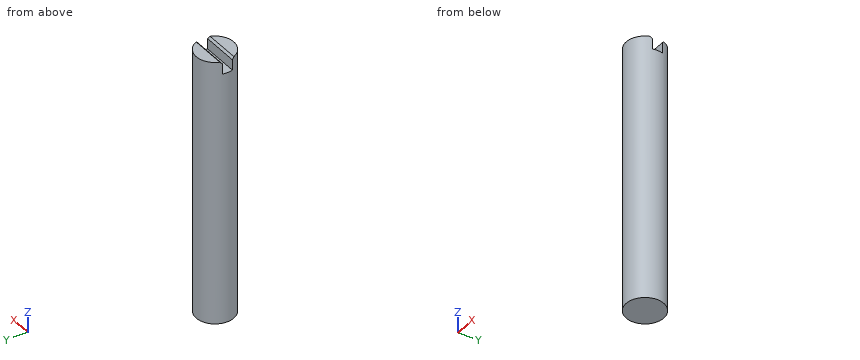
```python
from build123d import *

# Parameters (mm, degrees)
SKETCH1_R           = 4.7625
BOSS_EXTRUDE1_DEPTH = 67.6402
SKETCH2_W           = 9.525
SKETCH2_H           = 2.54
CUT_EXTRUDE1_DEPTH  = 3.175
CHAMFER1_SIZE       = 0.508


with BuildPart() as part:
    # Sketch1 → Boss-Extrude1 (new body)
    with BuildSketch(Plane.XY):
        Circle(SKETCH1_R)
    extrude(amount=-BOSS_EXTRUDE1_DEPTH)

    # Sketch2 → Cut-Extrude1 (cut)
    with BuildSketch(Plane.XY):
        Rectangle(SKETCH2_W, SKETCH2_H)
    extrude(amount=-CUT_EXTRUDE1_DEPTH, mode=Mode.SUBTRACT)

    # Chamfer1
    chamfer1_edges = [part.edges().sort_by_distance(p)[0] for p in [
        (0, -1.27, 0),
        (0, 1.27, 0),
    ]]
    chamfer(chamfer1_edges, length=CHAMFER1_SIZE)


solid = part.part
```
Check sheet for the modelled part. Datum: model origin and axes. Units: mm. Coordinates: 2 decimals unless noted, no trailing zeros. Order: outer loops, then holes, each group sorted by start corner. A loop starts at its lowest first (then second) coordinate and runs counter-clockwise, first axis right, second up. Notation, with made-up numbers: M 52.5,10 L 83.5,10 A9 ccw 83.5,16 Z; hole C 71.25,-38.5 d6. An arc over 180 degrees is marked long. Write each question's results on one line, items separated by ' | '. Start each with the question number.
1. Cross-section at C-C on y = 0. Record the cut outline in (x, z) (1 decimal), and give its area (3 significant figures).
2. Go/stop test with flat-tipped pins: P1, Ø3, axis at x = -3.5, z = -32, coming from the -Y side; P2, Ø1.3, axis at x = 0.5, y = 0, coming from the +Z side (3 decimals). Record where each tip stops, or that it passes through.
3. Cross-section at D-D on y = -2.75. Record the cut outline in (x, z).
4. Cross-section at B-B on z = -19. Record the cut outline in (x, y) (1 decimal), and give its area (3 significant figures).
5. Material ranges on probe 1 along Z at (x, y) = (0.5, 0.5) (3 decimals); probe 2 along X at (y, z) = (-0.25, -10); probe 3 along Y at (x, z) = (4.25, -56), recorded low to high.
6. Cross-section at A-A on x = -1.75. Record the cut outline in (y, z) (3 decimals).
Checks:
1) outline: M -4.8,-67.6 L 4.8,-67.6 L 4.8,-3.2 L -4.8,-3.2 Z | area: 614 mm²
2) P1: stops at y = -4.32 | P2: stops at z = -3.175
3) outline: M -3.89,-67.64 L 3.89,-67.64 L 3.89,0 L -3.89,0 Z
4) outline: C 0,0 d9.5 | area: 71.3 mm²
5) probe 1: z = -67.64 to -3.175 | probe 2: x = -4.76 to 4.76 | probe 3: y = -2.15 to 2.15
6) outline: M -4.429,-67.64 L 4.429,-67.64 L 4.429,0 L 1.778,0 L 1.27,-0.508 L 1.27,-3.175 L -1.27,-3.175 L -1.27,-0.508 L -1.778,0 L -4.429,0 Z
